Autodesk Inventor part; units mm, degrees
ref_plane "YZ Plane" through (0, 0, 0) normal (1, 0, 0) x (0, 1, 0)
ref_plane "XZ Plane" through (0, 0, 0) normal (0, 1, 0) x (-1, 0, 0)
ref_plane "XY Plane" through (0, 0, 0) normal (0, 0, 1) x (1, 0, 0)
sketch "Sketch1" plane through (0, 0, 0) normal (0, 1, 0) x (-1, 0, 0)
  line L0 (0, 0) -> (4, 0)
  line L1 (4, 0) -> (4, -32)
  line L2 (4, -32) -> (0, -32)
  line L3 (0, -32) -> (0, 0)
  dimension "d0" = 4
  dimension "d1" = 32
extrude "Extrusion1" add sketch "Sketch1" along normal blind 1
fillet "Fillet1" radius 2 4 edges at (0, 0.5, 0) (-4, 0.5, 0) (0, 0.5, -32) (-4, 0.5, -32)
sketch "Sketch2" plane through (0, 1, 0) normal (0, 1, 0) x (1, 0, 0)
  circle A0 centre (-2, 16) radius 3.5
  arc A1 (-4, 2) -> (0, 2) centre (-2, 2) ccw
  line L0 (0, 2) -> (0, 30)
  point P0 (0, 0)
  point P1 (-2, 0)
  dimension "d5" = 7
  dimension "d6" = 16
  dimension "d7" = 2
extrude "Extrusion2" add sketch "Sketch2" along normal blind 3
sketch "Sketch3" plane through (0, 1, 0) normal (0, -1, 0) x (1, 0, 0)
  line L0 (0, -13.1277) -> (0, -18.8723)
  arc A0 (0, -18.8723) -> (0, -13.1277) centre (-2, -16) ccw
  line L1 (-4, -18.8723) -> (-4, -13.1277)
  arc A1 (-4, -13.1277) -> (-4, -18.8723) centre (-2, -16) ccw
  arc A2 (0, -18.8723) -> (0, -13.1277) centre (-2, -16) ccw
  arc A3 (-4, -13.1277) -> (-4, -18.8723) centre (-2, -16) ccw
  line L2 (-4, -13.1277) -> (-4, -18.8723)
  line L3 (-4, -30) -> (-4, -2)
  line L4 (0, -13.1277) -> (0, -18.8723)
  line L5 (0, -2) -> (0, -30)
  point P0 (0, 0)
extrude "Extrusion3" add sketch "Sketch3" along normal blind 1
sketch "Sketch4" plane through (0, 0, 0) normal (0, -1, 0) x (1, 0, 0)
  arc A0 (-4, -30) -> (0, -30) centre (-2, -30) ccw
  line L0 (0, -18.8723) -> (0, -30)
  arc A1 (0, -18.8723) -> (0, -13.1277) centre (-2, -16) ccw
  line L1 (0, -2) -> (0, -13.1277)
  arc A2 (0, -2) -> (-4, -2) centre (-2, -2) ccw
  line L2 (-4, -13.1277) -> (-4, -2)
  arc A3 (-4, -13.1277) -> (-4, -18.8723) centre (-2, -16) ccw
  line L3 (-4, -30) -> (-4, -18.8723)
  circle A4 centre (-2, -16) radius 1
  point P0 (0, 0)
  dimension "d12" = 2
extrude "Extrusion4" cut sketch "Sketch4" against normal through all contours A4
sketch "Sketch5" plane through (-2, 4, -16) normal (0, 1, 0) x (1, 0, 0)
  circle A0 centre (0, 0) radius 1
  circle A1 centre (0, 0) radius 2.5
  point P0 (2, -16)
  dimension "d15" = 5
extrude "Extrusion5" cut sketch "Sketch5" against normal blind 3
sketch "Sketch6" plane through (0, 0, 0) normal (0, -1, 0) x (1, 0, 0)
  circle A0 centre (-2, -8) radius 1
  circle A1 centre (-2, -24) radius 1
  circle A2 centre (-2, -16) radius 1
  point P0 (0, 0)
  dimension "d18" = 2
  dimension "d19" = 2
  dimension "d20" = 16
  dimension "d21" = 8
extrude "Extrusion6" cut sketch "Sketch6" against normal through all contours A0 | A1
properties part number "ServoWings"
Input: part model. Units: mm. Frame: model coordinates. A direction names the side the tool comes from. Coordinates: 2 decimals unless noted, no trailing zeros. Write each loop counter-clockwise with the first axis right and the second up, starting at its lowest first coordinate (ties: lowest second). Pieces come first, ordered by that corner, then holes. Notation, with made-up numbers: M 19.5,56.25 L 23.5,56.25 A13 ccw 23.5,60.25 Z; hole C 22.5,46 d7. An arc over 180 degrees is marked long. Use one line per item in the form item = value.
Q1. Draft query along X for faces 5 (the face through (-2.13, 0.49, -7.01)), 6 (the face through (1.233, 2.479, -17.341)), 7 (the face through (-0.6, 0.51, -0.57)). Return one class per face: released by +X, released by -X, zero draft, split by the parting line, or undercut.
Answer below:
face_5 = undercut
face_6 = split by the parting line
face_7 = released by +X
Q2. Set-up query: faces 1 (the face through (-4, 0.5, -7.5)), 2 (the face through (-1, 1, -15)), 3 (the face through (-5.5, 0.5, -16)), 4 (the face through (0, 0.5, -7.6)). Return all of +Z, -Z, +X, -X, +Y, -Y with unobstructed straight access to the full face (end or side cutting, diameter ignored); none if empty.
Answer below:
face_1 = +Z, -X, +Y, -Y
face_2 = +Y
face_3 = -X, +Y, -Y
face_4 = +Z, +X, +Y, -Y
Q3. Section C-C (y = 3.55). Return loops of the section in (x, z), plus the area to 3 significant figures.
Answer below:
outline = C -2,-16 d7; hole C -2,-16 d5
area = 18.8 mm²
Q4. Material intervals for probe 1 along Z at (x, y) = (-2, 0.55); probe 2 along Y at (x, z) = (-1, -18); probe 3 along Z at (x, y) = (-0.5, 1.65), sorted ascending. Write a range as from..to.
Answer below:
probe_1 = -32..-25, -23..-17, -15..-9, -7..0
probe_2 = 0..1
probe_3 = -19.16..-18, -14..-12.84
Q5. First-contact query: pin 1 (4 mm diameter, centred on x = -2, z = -17, fed in from +Y); pin 2 (1.2 mm diameter, centred on x = -3, z = -22.5, fed in from +Y); pin 3 (0.8 mm diameter, centred on y = 0.5, z = -8.5, fed in from -X); pin 4 (1.1 mm diameter, centred on y = 0.5, z = -9.5, fed in from +X). Flat tips, straight axial feed; report the tip coordinate or a pass-through.
Answer below:
pin_1 = 4
pin_2 = 1
pin_3 = -4
pin_4 = 0
Q6. Section D-D (x = -3.5). Return loops of the section in (y, z).
Answer below:
outline = M 0,-31.32 L 1,-31.32 L 1,-19.16 L 4,-19.16 L 4,-18 L 1,-18 L 1,-14 L 4,-14 L 4,-12.84 L 1,-12.84 L 1,-0.68 L 0,-0.68 Z
Q7. Section A-A (z = -8). Return loops of the section in (x, y), plus the area to 3 significant figures.
Answer below:
outline = M -4,0 L -3,0 L -3,1 L -4,1 Z; M -1,0 L 0,0 L 0,1 L -1,1 Z
area = 2.00 mm²
Q8. Section B-B (y = 0.55). Count the separate pieces of the cut face and the enclosed holes in it, plus the area to 3 significant figures.
Answer below:
separate_pieces = 1
enclosed_holes = 3
area = 127 mm²
